Here's how the part is built. I have some questions about the finished solid (model axes, mm). A direction names the side the tool comes from. Round coordinates to 2 decimals unless told otherwise and drop trailing zeros. Write each loop counter-clockwise with the first axis right and the second up, starting at its lowest first coordinate (ties: lowest second). Pieces come first, ordered by that corner, then holes. Notation, with made-up numbers: (36, -14) -> (44, -14) arc R26 ccw to (44, 13) -> close; hole circle Ø6 at (0.25, 39.25). An arc over 180 degrees is marked (long way). Answer in a Markdown table with one row per item.
from build123d import *

# Parameters (mm, degrees)
SCHIZZO1_R                   = 22.5
ESTRUSIONE_ESTRUSIONE1_DEPTH = 35.8
SCHIZZO2_R                   = 13
ESTRUSIONE_ESTRUSIONE3_DEPTH = 14
SCHIZZO3_R                   = 16
ESTRUSIONE_ESTRUSIONE4_DEPTH = 9
SCHIZZO4_W                   = 18
SCHIZZO4_H                   = 6
ESTRUSIONE_ESTRUSIONE5_DEPTH = 25.1


with BuildPart() as part:
    # Schizzo1 → Estrusione-Estrusione1 (new body)
    with BuildSketch(Plane(origin=(0, 0, 0), x_dir=(1, 0, 0), z_dir=(0, 1, 0))):
        Circle(SCHIZZO1_R)
    extrude(amount=ESTRUSIONE_ESTRUSIONE1_DEPTH)

    # Schizzo2 → Estrusione-Estrusione3 (add)
    with BuildSketch(Plane(origin=(0, 35.8, 0), x_dir=(1, 0, 0), z_dir=(0, 1, 0))):
        Circle(SCHIZZO2_R)
    extrude(amount=ESTRUSIONE_ESTRUSIONE3_DEPTH)

    # Schizzo3 → Estrusione-Estrusione4 (add)
    with BuildSketch(Plane(origin=(0, 49.8, 0), x_dir=(1, 0, 0), z_dir=(0, 1, 0))):
        Circle(SCHIZZO3_R)
    extrude(amount=ESTRUSIONE_ESTRUSIONE4_DEPTH)

    # Schizzo4 → Estrusione-Estrusione5 (add)
    with BuildSketch(Plane(origin=(0, 58.8, 0), x_dir=(1, 0, 0), z_dir=(0, 1, 0))):
        Rectangle(SCHIZZO4_W, SCHIZZO4_H)
    extrude(amount=ESTRUSIONE_ESTRUSIONE5_DEPTH)


solid = part.part
1) I want a section at C-C, the plane y = 53. List the corners of the cut face in (x, z) for me, and give its area (3 significant figures).
Response:
| item | result |
|---|---|
| outline | circle Ø32 at (0, 0) |
| area | 804 mm^2 |
2) I want a section at D-D, the plane z = 9. List the corners of the cut face in (x, y) for me.
Response:
| item | result |
|---|---|
| outline | (-20.62, 0) -> (20.62, 0) -> (20.62, 35.8) -> (9.38, 35.8) -> (9.38, 49.8) -> (13.23, 49.8) -> (13.23, 58.8) -> (-13.23, 58.8) -> (-13.23, 49.8) -> (-9.38, 49.8) -> (-9.38, 35.8) -> (-20.62, 35.8) -> close |
3) We'd pull the mould along Y, two halves only. Please class faces 4 (the face through (0, 83.9, 0)), 5 (the face through (-9, 71, 0)), 6 (the face through (-1.3, 49.8, -13.1)): +Y half, -Y half, draft (parallel to the pull), parting line (faces both ways), or undercut.
Response:
| item | result |
|---|---|
| face 4 | +Y half |
| face 5 | draft |
| face 6 | undercut |
4) I want a section at B-B, the plane x = 0. List the corners of the cut face in (y, z) for me, and give its area (3 significant figures).
Response:
| item | result |
|---|---|
| outline | (0, -22.5) -> (35.8, -22.5) -> (35.8, -13) -> (49.8, -13) -> (49.8, -16) -> (58.8, -16) -> (58.8, -3) -> (83.9, -3) -> (83.9, 3) -> (58.8, 3) -> (58.8, 16) -> (49.8, 16) -> (49.8, 13) -> (35.8, 13) -> (35.8, 22.5) -> (0, 22.5) -> close |
| area | 2,410 mm^2 |
5) I want a section at A-A, the plane z = 0. List the corners of the cut face in (x, y) for me, and give its area (3 significant figures).
Response:
| item | result |
|---|---|
| outline | (-22.5, 0) -> (22.5, 0) -> (22.5, 35.8) -> (13, 35.8) -> (13, 49.8) -> (16, 49.8) -> (16, 58.8) -> (9, 58.8) -> (9, 83.9) -> (-9, 83.9) -> (-9, 58.8) -> (-16, 58.8) -> (-16, 49.8) -> (-13, 49.8) -> (-13, 35.8) -> (-22.5, 35.8) -> close |
| area | 2,710 mm^2 |
6) I need wall thicknesses on line 1 (Y direction, x = -13, z = 4); line 2 (Y direction, x = -14, z = -9); line 3 (Z direction, x = 0, y = 33.5). Which ranges of each line are inside material? Lowest first, please. Write a range as [from, to].
Response:
| item | result |
|---|---|
| line 1 | y = [0, 35.8], [49.8, 58.8] |
| line 2 | y = [0, 35.8] |
| line 3 | z = [-22.5, 22.5] |
7) Which directions (+Z, -Z, +X, -X, +Y, -Y) give clear straight access to the entire face, cutting with the end or side of a thin tool? Please do faces 1 (the face through (0, 71, -3)), 2 (the face through (10, 35.8, 10)), 3 (the face through (9, 71, 0)).
Response:
| item | result |
|---|---|
| face 1 | -Z, +X, -X, +Y |
| face 2 | none |
| face 3 | +Z, -Z, +X, +Y |
8) For pin 1 (1.5 mm diameter, centred on y = 50.5, z = -3, fed in from -X); pin 2 (20 mm diameter, centred on x = 3.5, y = 75.5, fed in from -Z); pin 3 (2 mm diameter, centred on x = -1.5, z = -12.5, fed in from +Y), each with a flat end and sliding along its axis, tell me the tip position at first contact or that it passes through.
Response:
| item | result |
|---|---|
| pin 1 | stops at x = -15.84 |
| pin 2 | stops at z = -3 |
| pin 3 | stops at y = 58.8 |
